The listing builds one solid part. Answer for the finished solid, in the listing's coordinates (mm). Give positions to 0.01 mm unless a question says otherwise; leave off trailing zeros. Write each loop counter-clockwise with the first axis right and the second up, starting at its lowest first coordinate (ties: lowest second). Pieces come first, ordered by that corner, then holes.
```python
from build123d import *

# Parameters (mm, degrees)
SKETCH4_R           = 28.575
BOSS_EXTRUDE2_DEPTH = 0.254
SKETCH5_R           = 15.875
CUT_EXTRUDE5_DEPTH  = 1.254
SKETCH6_R           = 4.699
CUT_EXTRUDE6_DEPTH  = 1.254
CUT_EXTRUDE11_DEPTH = 1.254


with BuildPart() as part:
    # Sketch4 → Boss-Extrude2 (new body)
    with BuildSketch(Plane.XY):
        Circle(SKETCH4_R)
    extrude(amount=BOSS_EXTRUDE2_DEPTH)

    # Sketch5 → Cut-Extrude5 (cut, through all)
    with BuildSketch(Plane.XY.offset(0.254)):
        Circle(SKETCH5_R)
    extrude(amount=-CUT_EXTRUDE5_DEPTH, mode=Mode.SUBTRACT)

    # Sketch6 → Cut-Extrude6 (cut, through all)
    with BuildSketch(Plane.XY.offset(0.254)):
        with Locations((22.225, 0)):
            Circle(SKETCH6_R)
        with BuildLine():
            ThreePointArc((19.03814289, -19.038143063), (19.038142992, -12.392753462), (12.392753391, -12.392753504))
            ThreePointArc((12.392753391, -12.392753504), (6.706909655, -16.191912762), (-3.11e-07, -17.526))
            ThreePointArc((-3.11e-07, -17.526), (-4.699, -22.224999917), (-4.77e-07, -26.924))
            ThreePointArc((-4.77e-07, -26.924), (10.303368456, -24.874532648), (19.03814289, -19.038143063))
        make_face()
        with BuildLine():
            ThreePointArc((-19.038143063, -19.03814289), (-12.392753462, -19.038142992), (-12.392753504, -12.392753391))
            ThreePointArc((-12.392753504, -12.392753391), (-16.191912762, -6.706909655), (-17.526, 3.11e-07))
            ThreePointArc((-17.526, 3.11e-07), (-22.224999917, 4.699), (-26.924, 4.77e-07))
            ThreePointArc((-26.924, 4.77e-07), (-24.874532648, -10.303368456), (-19.038143063, -19.03814289))
        make_face()
        with BuildLine():
            ThreePointArc((-19.03814289, 19.038143063), (-19.038142992, 12.392753462), (-12.392753391, 12.392753504))
            ThreePointArc((-12.392753391, 12.392753504), (-6.706909655, 16.191912762), (3.11e-07, 17.526))
            ThreePointArc((3.11e-07, 17.526), (4.699, 22.224999917), (4.77e-07, 26.924))
            ThreePointArc((4.77e-07, 26.924), (-10.303368456, 24.874532648), (-19.03814289, 19.038143063))
        make_face()
    extrude(amount=-CUT_EXTRUDE6_DEPTH, mode=Mode.SUBTRACT)

    # Sketch8 → Cut-Extrude11 (cut, through all)
    with BuildSketch(Plane.XY.offset(0.254)):
        with BuildLine():
            Line((11.748169406, 25.375786975), (9.518848094, 26.299202097))
            Line((9.518848094, 26.299202097), (9.751046558, 26.859778778))
            ThreePointArc((9.751046558, 26.859778778), (20.205576272, 20.205576272), (26.859778778, 9.751046558))
            Line((26.859778778, 9.751046558), (26.299202097, 9.518848094))
            Line((26.299202097, 9.518848094), (25.375786975, 11.748169406))
            Line((25.375786975, 11.748169406), (14.191115224, 7.115326676))
            ThreePointArc((14.191115224, 7.115326676), (11.225320151, 11.225320151), (7.115326676, 14.191115224))
            Line((7.115326676, 14.191115224), (11.748169406, 25.375786975))
        make_face()
        Polygon((-10.004856053, 27.472529104), (-12.351510066, 26.500513186), (-11.865502107, 25.327186179), (-9.518848094, 26.299202097), align=None)
        Polygon((-26.500513186, 12.351510066), (-27.472529104, 10.004856053), (-26.299202097, 9.518848094), (-25.327186179, 11.865502107), align=None)
        Polygon((-27.472529104, -10.004856053), (-26.500513186, -12.351510066), (-25.327186179, -11.865502107), (-26.299202097, -9.518848094), align=None)
        Polygon((-12.351510066, -26.500513186), (-10.004856053, -27.472529104), (-9.518848094, -26.299202097), (-11.865502107, -25.327186179), align=None)
        Polygon((10.004856053, -27.472529104), (12.351510066, -26.500513186), (11.865502107, -25.327186179), (9.518848094, -26.299202097), align=None)
        Polygon((26.500513186, -12.351510066), (27.472529104, -10.004856053), (26.299202097, -9.518848094), (25.327186179, -11.865502107), align=None)
    extrude(amount=-CUT_EXTRUDE11_DEPTH, mode=Mode.SUBTRACT)


solid = part.part
```
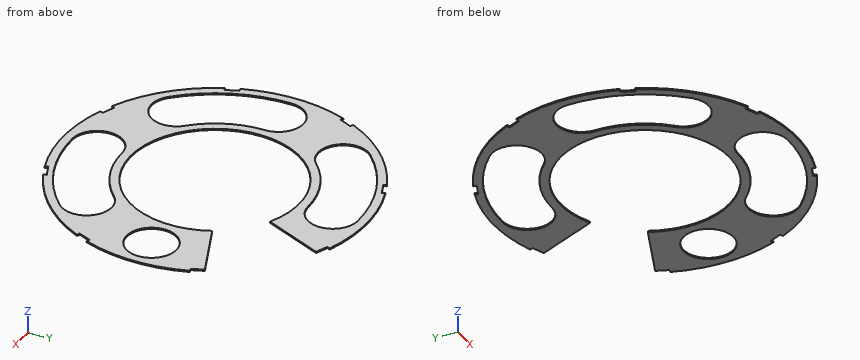
Item 1: A cutting plane is placed at B-B, the plane y = -7.5. Give the vertices of the cut face in (x, z), plus the area to 3 significant figures.
Conclusion:
outline: (-27.57, 0) - (-25.86, 0) - (-25.86, 0.25) - (-27.57, 0.25) - close; (-15.84, 0) - (-13.99, 0) - (-13.99, 0.25) - (-15.84, 0.25) - close; (13.99, 0) - (27.57, 0) - (27.57, 0.25) - (13.99, 0.25) - close
area: 4.35 mm2
Item 2: A cutting plane is placed at A-A, the plane y = -1.5. Give the vertices of the cut face in (x, z), plus the area to 3 significant figures.
Conclusion:
outline: (-28.54, 0) - (-26.88, 0) - (-26.88, 0.25) - (-28.54, 0.25) - close; (-17.46, 0) - (-15.8, 0) - (-15.8, 0.25) - (-17.46, 0.25) - close; (15.8, 0) - (17.77, 0) - (17.77, 0.25) - (15.8, 0.25) - close; (26.68, 0) - (28.54, 0) - (28.54, 0.25) - (26.68, 0.25) - close
area: 1.81 mm2
Item 3: A cutting plane is placed at C-C, the plane z = 0.05. Count the separate pieces of the cut face and the enclosed holes in it, plus the area to 3 significant figures.
Conclusion:
separate pieces: 1
enclosed holes: 4
area: 799 mm2
Item 4: Consider probe 1 along Y at (x, z) = (-9, 0.15); probe 2 along Y at (x, z) = (19.5, 0.1); probe 3 along Y at (x, z) = (-14, 0.15). Determine where each line is inside the solid, lowest interval first.
Conclusion:
probe 1: y = -27.12 to -13.08, 13.08 to 15.04, 25.38 to 27.12
probe 2: y = -20.89 to -18.5, -12.93 to -3.83, 3.83 to 9.31
probe 3: y = -24.91 to -20.09, -10.54 to -7.48, 7.48 to 11.34, 23 to 24.91
